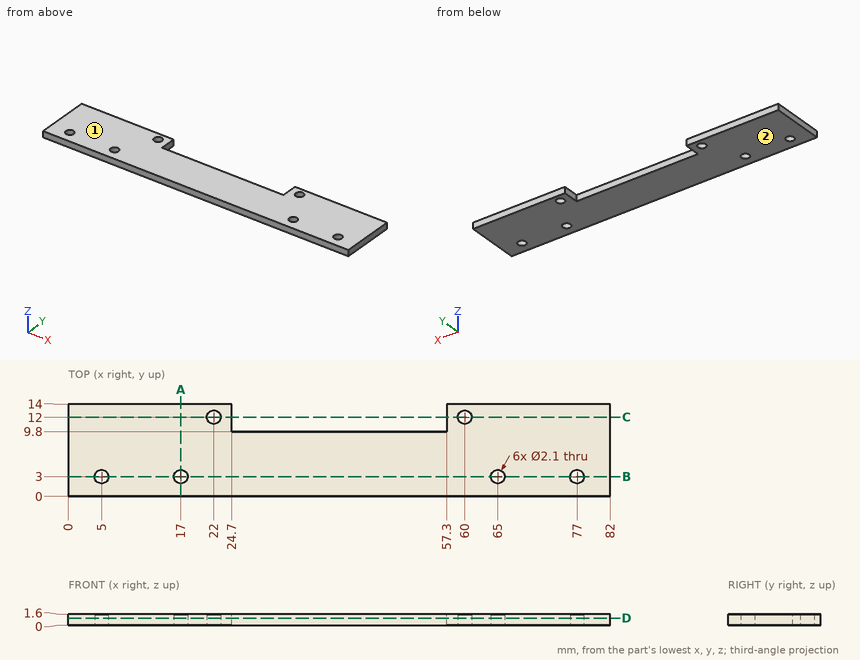
Could you check a few things on this drawing? It's one solid part, dimensions in mm from its lowest x, y, z. Coordinates: 2 decimals unless noted, no trailing zeros. Write each loop counter-clockwise with the first axis right and the second up, starting at its lowest first coordinate (ties: lowest second). Pieces come first, ordered by that corner, then holes. Notation, with made-up numbers: (-4.75, 45.5) - (44.25, 45.5) arc R24 ccw to (44.25, 83.5) - close; hole circle Ø3 at (41, 40). An arc over 180 degrees is marked (long way). Put each result on its own line as item: value. Start each with the question number.
Q1. Thinking about a two-plate mould opening in Z: for the marked faces 1 and 2, which applies, pulls with the +Z half, pulls with the -Z half, needs draft (parallel to the pull), parting line crosses it, or undercut?
Q2. I'm going to push flat-ended pins straight in: P1, Ø0.8, axis at x = 40, z = 0.5, coming from the +Y side; P2, Ø0.8, axis at y = 12, z = 0.5, coming from the -X side. Where does each tip first touch, or does it pass through?
Q3. I want a section at D-D on z = 1.05. Write out the boundary of the cut face in (x, y).
Q4. I want a section at B-B on y = 3. Write out the boundary of the cut face in (x, z), plus the area to 3 significant figures.
Q5. I want a section at A-A on x = 17. Write out the boundary of the cut face in (y, z), plus the area to 3 significant figures.
Q6. Please list where these lines run through material, in increasing order: L1, parallel to X at y = 3, z = 1.15; L2, parallel to X at y = 12, z = 0.15; L3, parallel to Y at x = 60, z = 0.95.
Q7. I want a section at C-C on y = 12. Write out the boundary of the cut face in (x, z).
Checks:
1. face 1: pulls with the +Z half
1. face 2: pulls with the -Z half
2. P1: y = 9.8
2. P2: x = 0
3. outline: (0, 0) - (82, 0) - (82, 14) - (57.3, 14) - (57.3, 9.8) - (24.7, 9.8) - (24.7, 14) - (0, 14) - close; hole circle Ø2.1 at (5, 3); hole circle Ø2.1 at (17, 3); hole circle Ø2.1 at (22, 12); hole circle Ø2.1 at (60, 12); hole circle Ø2.1 at (65, 3); hole circle Ø2.1 at (77, 3)
4. outline: (0, 0) - (3.95, 0) - (3.95, 1.6) - (0, 1.6) - close; (6.05, 0) - (15.95, 0) - (15.95, 1.6) - (6.05, 1.6) - close; (18.05, 0) - (63.95, 0) - (63.95, 1.6) - (18.05, 1.6) - close; (66.05, 0) - (75.95, 0) - (75.95, 1.6) - (66.05, 1.6) - close; (78.05, 0) - (82, 0) - (82, 1.6) - (78.05, 1.6) - close
4. area: 118 mm²
5. outline: (0, 0) - (1.95, 0) - (1.95, 1.6) - (0, 1.6) - close; (4.05, 0) - (14, 0) - (14, 1.6) - (4.05, 1.6) - close
5. area: 19.0 mm²
6. L1: 0 to 3.95, 6.05 to 15.95, 18.05 to 63.95, 66.05 to 75.95, 78.05 to 82
6. L2: 0 to 20.95, 23.05 to 24.7, 57.3 to 58.95, 61.05 to 82
6. L3: 0 to 10.95, 13.05 to 14
7. outline: (0, 0) - (20.95, 0) - (20.95, 1.6) - (0, 1.6) - close; (23.05, 0) - (24.7, 0) - (24.7, 1.6) - (23.05, 1.6) - close; (57.3, 0) - (58.95, 0) - (58.95, 1.6) - (57.3, 1.6) - close; (61.05, 0) - (82, 0) - (82, 1.6) - (61.05, 1.6) - close
